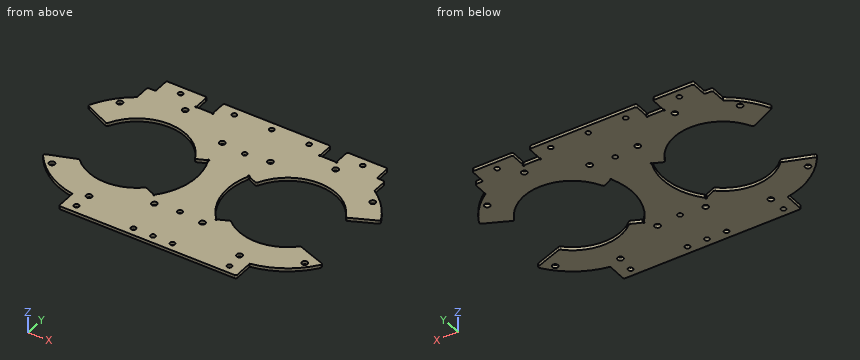
```python
from build123d import *

# Parameters (mm, degrees)
SKETCH_1_R          = 1.5
SKETCH_1_R_2        = 1.75
EXTRUDE_1_DEPTH     = 2
CUT_EXTRUDE_3_DEPTH = 10
SKETCH_2_R          = 0.5
CUT_EXTRUDE_1_DEPTH = 10
SKETCH_8_W          = 5
SKETCH_8_H          = 10.1
CUT_EXTRUDE_4_DEPTH = 10
FILLET_2_R          = 1


with BuildPart() as part:
    # 草图1 → 凸台-拉伸1 (new body)
    with BuildSketch(Plane.XY):
        with BuildLine():
            Line((-54.5, -47.539457296), (-54.5, -60))
            Line((-54.5, -60), (54.5, -60))
            Line((54.5, -60), (54.5, -47.539457296))
            ThreePointArc((54.5, -47.539457296), (72.332250623, -40.592840532), (86.061310432, -27.260265254))
            Line((86.061310432, -27.260265254), (67.983033669, -20.680310625))
            ThreePointArc((67.983033669, -20.680310625), (16.643405824, 4.842476776), (73.439233611, 12.678547852))
            Line((73.439233611, 12.678547852), (89.979350725, 20.391331129))
            ThreePointArc((89.979350725, 20.391331129), (82.849108186, 31.441497738), (73, 40.155946011))
            Line((73, 40.155946011), (73, 60))
            Line((73, 60), (43.1, 60))
            Line((43.1, 60), (43.1, 49.9))
            Line((43.1, 49.9), (32.9, 49.9))
            Line((32.9, 49.9), (32.9, 60))
            Line((32.9, 60), (-32.9, 60))
            Line((-32.9, 60), (-32.9, 49.9))
            Line((-32.9, 49.9), (-43.1, 49.9))
            Line((-43.1, 49.9), (-43.1, 60))
            Line((-43.1, 60), (-73, 60))
            Line((-73, 60), (-73, 40.155946011))
            ThreePointArc((-73, 40.155946011), (-82.849108186, 31.441497738), (-89.979350725, 20.391331129))
            Line((-89.979350725, 20.391331129), (-73.439233611, 12.678547852))
            ThreePointArc((-73.439233611, 12.678547852), (-16.643405824, 4.842476776), (-67.983033669, -20.680310625))
            Line((-67.983033669, -20.680310625), (-86.061310432, -27.260265254))
            ThreePointArc((-86.061310432, -27.260265254), (-72.332250623, -40.592840532), (-54.5, -47.539457296))
        make_face()
        with Locations((-47, -55)):
            Circle(SKETCH_1_R, mode=Mode.SUBTRACT)
        with Locations((-77.716251763, -31.466251763)):
            Circle(SKETCH_1_R_2, mode=Mode.SUBTRACT)
        with Locations((-46.25, -44.5)):
            Circle(SKETCH_1_R_2, mode=Mode.SUBTRACT)
        with Locations((-12, -55)):
            Circle(SKETCH_1_R, mode=Mode.SUBTRACT)
        with Locations((-14.783748237, -31.466251763)):
            Circle(SKETCH_1_R_2, mode=Mode.SUBTRACT)
        with Locations((0, -55)):
            Circle(SKETCH_1_R, mode=Mode.SUBTRACT)
        with Locations((12, -55)):
            Circle(SKETCH_1_R, mode=Mode.SUBTRACT)
        with Locations((0, -30)):
            Circle(SKETCH_1_R, mode=Mode.SUBTRACT)
        with Locations((14.783748237, -31.466251763)):
            Circle(SKETCH_1_R_2, mode=Mode.SUBTRACT)
        with Locations((47, -55)):
            Circle(SKETCH_1_R, mode=Mode.SUBTRACT)
        with Locations((46.25, -44.5)):
            Circle(SKETCH_1_R_2, mode=Mode.SUBTRACT)
        with Locations((77.716251763, -31.466251763)):
            Circle(SKETCH_1_R_2, mode=Mode.SUBTRACT)
        with Locations((-77.716251763, 31.466251763)):
            Circle(SKETCH_1_R_2, mode=Mode.SUBTRACT)
        with Locations((-46.25, 44.5)):
            Circle(SKETCH_1_R_2, mode=Mode.SUBTRACT)
        with Locations((-56, 55)):
            Circle(SKETCH_1_R, mode=Mode.SUBTRACT)
        with Locations((-14.783748237, 31.466251763)):
            Circle(SKETCH_1_R_2, mode=Mode.SUBTRACT)
        with Locations((-23, 55)):
            Circle(SKETCH_1_R, mode=Mode.SUBTRACT)
        with Locations((0, 30)):
            Circle(SKETCH_1_R, mode=Mode.SUBTRACT)
        with Locations((14.783748237, 31.466251763)):
            Circle(SKETCH_1_R_2, mode=Mode.SUBTRACT)
        with Locations((0, 55)):
            Circle(SKETCH_1_R, mode=Mode.SUBTRACT)
        with Locations((23, 55)):
            Circle(SKETCH_1_R, mode=Mode.SUBTRACT)
        with Locations((46.25, 44.5)):
            Circle(SKETCH_1_R_2, mode=Mode.SUBTRACT)
        with Locations((77.716251763, 31.466251763)):
            Circle(SKETCH_1_R_2, mode=Mode.SUBTRACT)
        with Locations((56, 55)):
            Circle(SKETCH_1_R, mode=Mode.SUBTRACT)
    extrude(amount=EXTRUDE_1_DEPTH)

    # 草图7 → 切除-拉伸3 (cut)
    with BuildSketch(Plane.XY.offset(2)):
        with BuildLine():
            Line((19.156748699, -25.198327999), (26.012492454, -22.145954221))
            ThreePointArc((26.012492454, -22.145954221), (16.882810612, -6.129289311), (18.843636271, 12.202099292))
            Line((18.843636271, 12.202099292), (12.448818067, 15.049255794))
            ThreePointArc((12.448818067, 15.049255794), (9.753424818, -6.08276253), (19.156748699, -25.198327999))
        make_face()
    cut_extrude_3 = extrude(amount=-CUT_EXTRUDE_3_DEPTH, mode=Mode.SUBTRACT)

    # 镜向2: 切除-拉伸3 across plane
    add(cut_extrude_3.mirror(Plane(origin=(0, 0, 0), x_dir=(0, 0, 1), z_dir=(1, 0, 0))), mode=Mode.SUBTRACT)

    # 草图2 → 切除-拉伸1 (cut)
    with BuildSketch(Plane.XY.offset(2)):
        with Locations((-43.1, 49.9)):
            Circle(SKETCH_2_R)
        with Locations((-32.9, 49.9)):
            Circle(SKETCH_2_R)
        with Locations((32.9, 49.9)):
            Circle(SKETCH_2_R)
        with Locations((43.1, 49.9)):
            Circle(SKETCH_2_R)
        with Locations((-12.448818067, 15.049255794)):
            Circle(SKETCH_2_R)
        with Locations((12.448818067, 15.049255794)):
            Circle(SKETCH_2_R)
        with Locations((-19.156748699, -25.198327999)):
            Circle(SKETCH_2_R)
        with Locations((19.156748699, -25.198327999)):
            Circle(SKETCH_2_R)
    extrude(amount=-CUT_EXTRUDE_1_DEPTH, mode=Mode.SUBTRACT)

    # 草图8 → 切除-拉伸4 (cut)
    with BuildSketch(Plane(origin=(0, 0, 0), x_dir=(-1, 0, 0), z_dir=(0, 0, -1))):
        with Locations((70.5, 54.95)):
            Rectangle(SKETCH_8_W, SKETCH_8_H)
        with Locations((-70.5, 54.95)):
            Rectangle(SKETCH_8_W, SKETCH_8_H)
    extrude(amount=-CUT_EXTRUDE_4_DEPTH, mode=Mode.SUBTRACT)

    # 圆角2
    fillet_2_edges = [part.edges().sort_by_distance(p)[0] for p in [
        (18.843636271, 12.202099292, 1),
        (26.012492454, -22.145954221, 1),
        (-26.012492454, -22.145954221, 1),
        (-18.843636271, 12.202099292, 1),
        (-73, 49.9, 1),
        (68, 60, 1),
        (-68, 49.9, 1),
        (-68, 60, 1),
        (68, 49.9, 1),
        (73, 49.9, 1),
        (-67.983033669, -20.680310625, 1),
        (-73.439233611, 12.678547852, 1),
        (-89.979350725, 20.391331129, 1),
        (-43.1, 60, 1),
        (-32.9, 60, 1),
        (32.9, 60, 1),
        (43.1, 60, 1),
        (89.979350725, 20.391331129, 1),
        (73.439233611, 12.678547852, 1),
        (67.983033669, -20.680310625, 1),
        (86.061310432, -27.260265254, 1),
        (54.5, -60, 1),
        (-54.5, -60, 1),
        (-86.061310432, -27.260265254, 1),
    ]]
    fillet(fillet_2_edges, radius=FILLET_2_R)


solid = part.part
```
Source: CAD feature listing. Evaluate the final solid. Frame: model axes, mm. Round coordinates to 2 decimals unless told otherwise and drop trailing zeros. Loops run counter-clockwise (first coordinate to the right, second up) from the corner with the lowest first, then second, coordinate; pieces in that order, holes last.
1. Ray query, L1, parallel to Y at x = 23.5, z = 0.35; L2, parallel to Y at x = 77, z = 1.3; L3, parallel to Y at x = -22.5, z = 1.7. Return the intervals inside material, ascending.
2. Section query B-B on y = -11. Output: boundary loops of the cut face in (x, z).
3. Section query A-A on z = 1.3. Give the number of separate pieces and of enclosed holes in the cut face, and give its area (3 significant figures).
4. Section query C-C on y = -38.5. Output: boundary loops of the cut face in (x, z), and give its area (3 significant figures).
Answers below:
1. L1: y = -60 to -23.26, 19.56 to 53.59, 56.41 to 60
1. L2: y = -37.18 to -33.06, -29.87 to -23.96, 14.34 to 29.87, 33.06 to 37.18
1. L3: y = -60 to -23.71, 18.33 to 53.59, 56.41 to 60
2. outline: (-10.92, 0) - (10.92, 0) - (10.92, 2) - (-10.92, 2) - close
3. separate pieces: 1
3. enclosed holes: 24
3. area: 11,100 mm2
4. outline: (-75.33, 0) - (75.33, 0) - (75.33, 2) - (-75.33, 2) - close
4. area: 301 mm2
